from build123d import *

# Parameters (mm, degrees)
EXTRUDE1_DEPTH     = 350
EXTRUDE1_2_DEPTH   = 350
EXTRUDE2_START     = -220
EXTRUDE2_DEPTH     = 1300
SKETCH3_W          = 220
SKETCH3_H          = 350
SKETCH4_W          = 220
SKETCH4_H          = 350
CUT_EXTRUDE1_DEPTH = 351.0000001


with BuildPart() as part:
    # Sketch1 → Extrude1 (new body)
    with BuildSketch(Plane.XY):
        Polygon((220, 850), (220, 1100), (0, 1100), (0, 0), (220, 0), (220, 350), (320, 600), align=None)
    extrude(amount=EXTRUDE1_DEPTH)



with BuildPart() as body_2:
    # Sketch1 → Extrude1 2 (new body)
    with BuildSketch(Plane.XY):
        Polygon((1740, 0), (1520, 0), (1520, 350), (1420, 600), (1520, 850), (1520, 1100), (1740, 1100), align=None)
    extrude(amount=EXTRUDE1_2_DEPTH)


with BuildPart() as part_1:
    add(part.part)

    add(body_2.part)  # Extrude2 merges body 2
    # Sketch2 → Extrude2 (add)
    with BuildSketch(Plane.ZY.offset(EXTRUDE2_START)):
        Polygon((50, 1050), (150, 1050), (300, 350), (50, 350), align=None)
    extrude(amount=-EXTRUDE2_DEPTH)

    # Sketch3 → Loft1 section 0
    with BuildSketch(Plane(origin=(0, 1100, 0), x_dir=(-1, 0, 0), z_dir=(0, 1, 0)), mode=Mode.PRIVATE) as loft1_s0:
        with Locations((-110, 175)):
            Rectangle(SKETCH3_W, SKETCH3_H)
    loft([loft1_s0.sketch, Vertex(110, 1350, 175)])

    # Sketch4 → Loft2 section 0
    with BuildSketch(Plane(origin=(0, 1100, 0), x_dir=(-1, 0, 0), z_dir=(0, 1, 0)), mode=Mode.PRIVATE) as loft2_s0:
        with Locations((-1630, 175)):
            Rectangle(SKETCH4_W, SKETCH4_H)
    loft([Vertex(1630, 1350, 175), loft2_s0.sketch])

    # Sketch7 → Cut-Extrude1 (cut, through all)
    with BuildSketch(Plane.XY):
        with BuildLine():
            Line((1520, 850), (1520, 1176.43317984))
            Line((1520, 1176.43317984), (220, 1176.43317984))
            Line((220, 1176.43317984), (220, 850))
            Line((220, 850), (420, 850))
            ThreePointArc((420, 850), (870, 1050), (1320, 850))
            Line((1320, 850), (1520, 850))
        make_face()
    extrude(amount=CUT_EXTRUDE1_DEPTH, mode=Mode.SUBTRACT)


solid = part_1.part
Work out the finished part from the listing and answer in its coordinate system (mm). A direction names the side the tool comes from. Coordinates: 2 decimals unless noted, no trailing zeros. Write each loop counter-clockwise with the first axis right and the second up, starting at its lowest first coordinate (ties: lowest second). Pieces come first, ordered by that corner, then holes. Notation, with made-up numbers: M 49,27.5 L 99,27.5 A18 cw 99,49.5 Z; hole C 21,71.25 d5. An arc over 180 degrees is marked long. Use one line per item in the form item = value. Start each with the question number.
1. The part is cut by section C-C (y = 1022). Give the vertices of the cut face in (x, z).
2. The part is cut by section B-B (z = 94.5). Give the vertices of the cut face in (x, y), plus the area to 3 significant figures.
3. Each of these flat-tipped pins is pushed along its axis until it touches: P1, Ø1, axis at x = 1079.5, y = 538.5, coming from the -Z side; P2, Ø1.5, axis at x = 1063.5, y = 501.5, coming from the +Z side. Where does it stop, or does it pass through?
4. The part is cut by section D-D (x = 166.5). Give the vertices of the cut face in (y, z).
5. The part is cut by section A-A (y = 1237). Give the vertices of the cut face in (x, z).
6. The mould has two halves that part along X. Classify faces 5 (the face through (0, 558, 173)), 6 (the face through (1618, 558, 350)), 7 (the face through (269.3, 473.25, 24.65)): released by +X, released by -X, zero draft, split by the parting line, or undercut.
7. Straight lines are drawn through the part: probe 1 along X at (y, z) = (949, 297); probe 2 along X at (y, z) = (865.5, 114.5); probe 3 along X at (y, z) = (880, 119). For each, find the intervals that lie inside material, in ascending order. Write a range as from..to.
8. A tool of negligible diameter and unlimited length cuts with its end or side. For faces 1 (the face through (1520, 173, 173)), 2 (the face through (270.7, 723.25, 24.65)), 3 (the face through (1562.008, 1195.472, 172.55)), 4 (the face through (1470.7, 473.25, 24.65)), from which of +Z, -Z, +X, -X, +Y, -Y can it reach the whole face along a straight path? Write none if from no direction.
Evaluation:
q1.outline = M 0,0 L 220,0 L 220,350 L 0,350 Z; M 687.88,50 L 1052.12,50 L 1052.12,156 L 687.88,156 Z; M 1520,0 L 1740,0 L 1740,350 L 1520,350 Z
q2.outline = M 0,0 L 220,0 L 220,350 L 1520,350 L 1520,0 L 1740,0 L 1740,1100 L 1680.6,1235 L 1579.4,1235 L 1520,1100 L 1520,850 L 1320,850 A606.25 ccw 420,850 L 220,850 L 220,1100 L 160.6,1235 L 59.4,1235 L 0,1100 Z
q2.area = 1,300,000 mm^2
q3.P1 = 50
q3.P2 = 267.7
q4.outline = M 0,0 L 1100,0 L 1221.59,85.11 L 1221.59,264.89 L 1100,350 L 0,350 Z
q5.outline = M 60.28,95.9 L 159.72,95.9 L 159.72,254.1 L 60.28,254.1 Z; M 1580.28,95.9 L 1679.72,95.9 L 1679.72,254.1 L 1580.28,254.1 Z
q6.face_5 = released by -X
q6.face_6 = zero draft
q6.face_7 = undercut
q7.probe_1 = 0..220, 1520..1740
q7.probe_2 = 0..220, 434.49..1305.51, 1520..1740
q7.probe_3 = 0..220, 449.02..1290.98, 1520..1740
q8.face_1 = +Z, -Z, -Y
q8.face_2 = -Z, +Y
q8.face_3 = +Z, -Z, +Y
q8.face_4 = -Z, -Y
